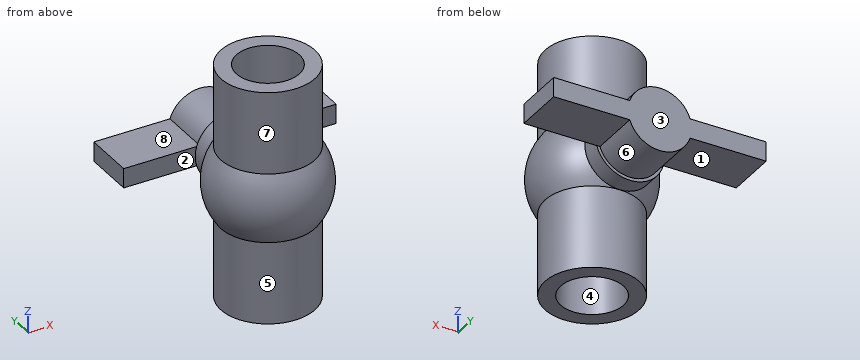
Autodesk Inventor part; units mm, degrees
ref_plane "Work Plane1" through (0, 15.7, 25.2827) normal (0, 1, 0) x (-1, 0, 0)
ref_plane "YZ Plane" through (0, 0, 0) normal (1, 0, 0) x (0, 1, 0)
ref_plane "XY Plane" through (0, 0, 0) normal (0, 0, 1) x (1, 0, 0)
sketch "Sketch1" plane through (0, 0, 0) normal (0, 1, 0) x (-1, 0, 0)
  line L0 (0, 0) -> (0, -39)
  line L1 (0, -39) -> (-15.7, -39)
  line L2 (-15.7, 39) -> (0, 39)
  line L3 (0, 39) -> (0, 0)
  arc A0 (-15.7, 11.5655) -> (-15.7, -11.5655) centre (0, 0) ccw
  line L4 (-15.7, -39) -> (-15.7, -11.5655)
  line L5 (-15.7, 11.5655) -> (-15.7, 39)
  dimension "d0" = 39
  dimension "d1" = 15.7
  dimension "d2" = 78
  dimension "d3" = 39
revolve "Revolution1" add sketch "Sketch1" angle 360 about axis through (0, 0, 0) along (0, 0, -1)
ref_plane "Work Plane1" through (0, 15.7, 25.2827) normal (0, 1, 0) x (-1, 0, 0)
split "Split1" plane through (0, 15.7, 25.2827) removes the side toward (0, 1, 0)
sketch "Sketch2" plane through (0, 15.7, 0) normal (0, 1, 0) x (1, 0, 0)
  circle A0 centre (0, 0) radius 11.5655
  line L0 (15.7, 11.5655) -> (-15.7, 11.5655)
  point P0 (0, 11.5655)
extrude "Extrusion1" add sketch "Sketch2" along normal blind 6
sketch "Sketch3" plane through (0, 0, 39) normal (0, 0, 1) x (1, 0, 0)
  circle A0 centre (0, 0) radius 10.5
  dimension "d7" = 21
extrude "Extrusion2" cut sketch "Sketch3" against normal blind 78
thread "Thread1"
sketch "Sketch4" plane through (0, 21.7, 0) normal (0, 1, 0) x (1, 0, 0)
  line L0 (35.4, -3.25) -> (35.4, 3.25)
  line L1 (-35.4, 3.25) -> (-35.4, -3.25)
  line L2 (35.4, 3.25) -> (10.0369, 3.25)
  line L3 (-10.0369, 3.25) -> (-35.4, 3.25)
  line L4 (-35.4, -3.25) -> (-10.0369, -3.25)
  line L5 (10.0369, -3.25) -> (35.4, -3.25)
  arc A0 (-10.0369, -3.25) -> (10.0369, -3.25) centre (0, 0) ccw
  arc A1 (10.0369, 3.25) -> (-10.0369, 3.25) centre (0, 0) ccw
  dimension "d12" = 70.8
  dimension "d13" = 6.5
extrude "Extrusion3" add sketch "Sketch4" along normal blind 17.1
properties part number "LlaveDesecho"
Input: part model. Units: mm. Frame: model coordinates. Face numbers are marked on the shaded views. A direction names the side the tool comes from. Give positions to 0.01 mm unless a question says otherwise; leave off trailing zeros. Write each loop counter-clockwise with the first axis right and the second up, starting at its lowest first coordinate (ties: lowest second). Pieces come first, ordered by that corner, then holes.
Q1. Material intervals for probe 1 along Y at (x, z) = (0, -22); probe 2 along Z at (x, y) = (10, 13); probe 3 along Z at (x, y) = (21, 22), sorted ascending.
Q2. Section C-C, the plane x = 5.5. Output: boundary loops of the cut face in (y, z), plus the area to 3 significant figures.
Q3. Section A-A, the plane y = 0. Output: boundary loops of the cut face in (x, z), plus the area to 3 significant figures.
Q4. Set-up query: the marked faces 5, 6, 7 and 8. Return all of +Z, -Z, +X, -X, +Y, -Y with unobstructed straight access to the full face (end or side cutting, diameter ignored); none if empty.
Q5. Section B-B, the plane z = 9.5. Output: boundary loops of the cut face in (x, y), plus the area to 3 significant figures.
Q6. Pull-direction query (Y, two-part tool) for the marked faces 1, 2, 3 and 4; classes: pulls with the +Y half, pulls with the -Y half, needs draft (parallel to the pull), parting line crosses it, or undercut.
Q7. First-contact query: P1, Ø2, axis at x = 7, z = -16, coming from the -Y side; P2, Ø13.5, axis at x = 23.5, y = 31.5, coming from the -Z side; P3, Ø4, axis at x = 5, y = 5.5, coming from the -Z side; P4, Ø12, axis at y = 23.5, z = 8.5, coming from the +X side. Flat tips, straight axial feed; report the tip coordinate or a pass-through.
Q8. Section D-D, the plane y = 35. Output: boundary loops of the cut face in (x, z).
Filled in:
1. probe 1: y = -15.7 to -10.5, 10.5 to 15.7
1. probe 2: z = -10.55 to 10.55
1. probe 3: z = -3.25 to 3.25
2. outline: (-14.71, -39) - (-8.94, -39) - (-8.94, 39) - (-14.71, 39) - (-14.71, 11.57) arc R18.71 ccw to (-14.71, -11.57) - close; (8.94, -39) - (14.71, -39) - (14.71, -11.57) arc R18.71 ccw to (15.7, -10.17) - (21.7, -10.17) - (21.7, -9) - (38.8, -9) - (38.8, 9) - (21.7, 9) - (21.7, 10.17) - (15.7, 10.17) arc R18.71 ccw to (14.71, 11.57) - (14.71, 39) - (8.94, 39) - close
2. area: 1,410 mm2
3. outline: (-15.7, -39) - (-10.5, -39) - (-10.5, 39) - (-15.7, 39) - (-15.7, 11.57) arc R19.5 ccw to (-15.7, -11.57) - close; (10.5, -39) - (15.7, -39) - (15.7, -11.57) arc R19.5 ccw to (15.7, 11.57) - (15.7, 39) - (10.5, 39) - close
3. area: 931 mm2
4. face 5: -Z
4. face 6: -Z, +Y
4. face 7: +Z
4. face 8: +Z, -X, +Y
5. outline: (-6.6, 15.7) arc R17.03 ccw (long way) to (6.6, 15.7) - (6.6, 21.7) - (4.59, 21.7) - (4.59, 38.8) - (-4.59, 38.8) - (-4.59, 21.7) - (-6.6, 21.7) - close; hole circle Ø21 at (0, 0)
5. area: 789 mm2
6. face 1: needs draft
6. face 2: undercut
6. face 3: pulls with the +Y half
6. face 4: undercut
7. P1: stops at y = -14.51
7. P2: stops at z = -3.25
7. P3: passes through
7. P4: stops at x = 35.4
8. outline: (-35.4, -3.25) - (-10.04, -3.25) arc R10.55 ccw to (10.04, -3.25) - (35.4, -3.25) - (35.4, 3.25) - (10.04, 3.25) arc R10.55 ccw to (-10.04, 3.25) - (-35.4, 3.25) - close
